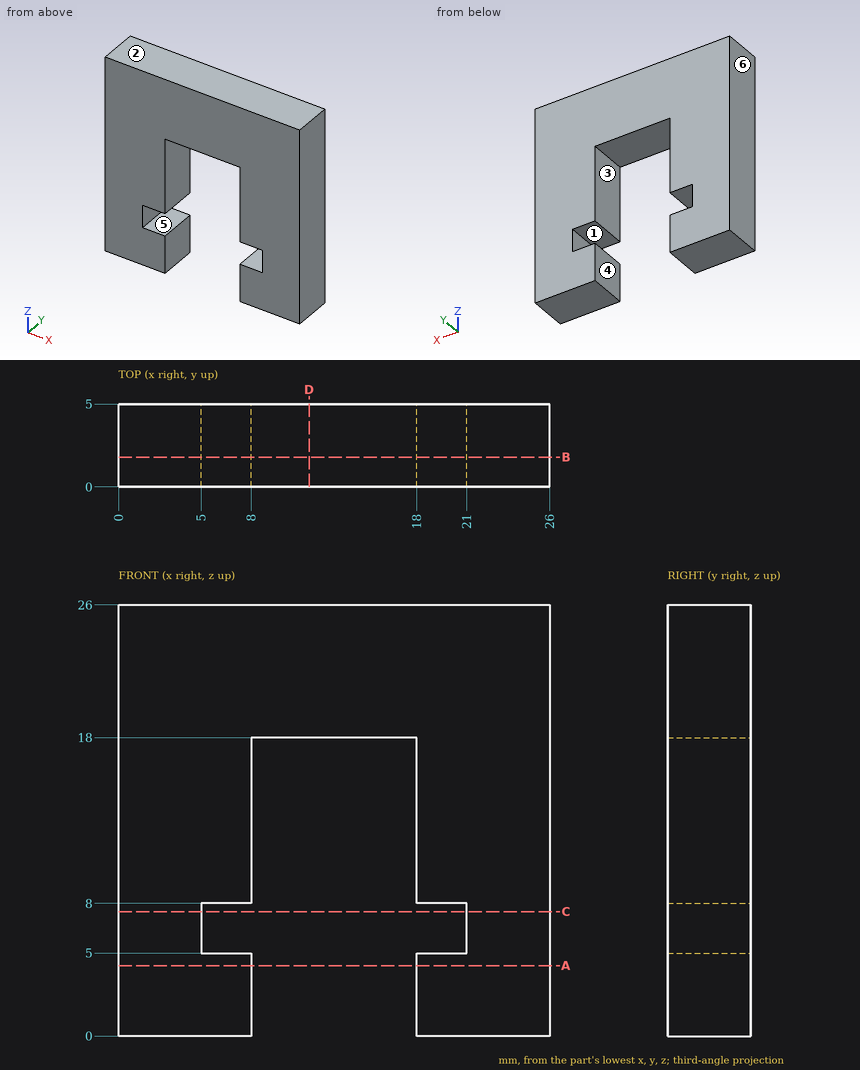
Geometry check sheet. Reference: drawing and pictorial views, mm from the part's lowest x, y, z. A direction names the side the tool comes from. Round coordinates to 2 decimals unless told otherwise and drop trailing zeros. Loops run counter-clockwise (first coordinate to the right, second up) from the corner with the lowest first, then second, coordinate; pieces in that order, holes last. Notation, with made-up numbers: M 46.25,-31 L 62.25,-31 A21 cw 62.25,-7 Z; hole C 12,89 d9. An arc over 180 degrees is marked long. Return JSON: item names as keys, results as strings. Group by question number.
(1) Section check B-B, the plane y = 1.8. Enter the section's corners in (x, z), and give its area (3 significant figures).
(2) Scan lines: line 1 along X through (y, z) = (0.7, 13.25); line 2 along X through (y, z) = (1.9, 6); line 3 along Z through (x, y) = (11, 0.2). Record each from-to range of solid material in increasing order. Write a range as [from, to].
(3) Section check A-A, the plane z = 4.25. Enter the section's corners in (x, y).
(4) Section check C-C, the plane z = 7.5. Enter the section's corners in (x, y), and give its area (3 significant figures).
(5) Set-up check for the marked faces 4, 5 and 6: record each of +Z, -Z, +X, -X, +Y, -Y from which the full face is reachable in a straight line by a thin tool's end or side.
(6) Go/stop test with a flat-tipped pin: pin 1 (1.5 mm diameter, centred on x = 12.5, y = 3, fed in from -Z). Record where the tip stops, or that it passes through.
(7) Section check D-D, the plane x = 11.5. Enter the section's corners in (y, z).
(8) Mould release check, pull along Z, two halves, no side actions. Record for the marked faces 1, 2 and 3: pulls with the +Z half, pulls with the -Z half, needs draft (parallel to the pull), parting line crosses it, or undercut.
Data:
{
 "1": {"outline": "M 0,0 L 8,0 L 8,5 L 5,5 L 5,8 L 8,8 L 8,18 L 18,18 L 18,8 L 21,8 L 21,5 L 18,5 L 18,0 L 26,0 L 26,26 L 0,26 Z", "area": "478 mm²"},
 "2": {"line 1": "[0, 8], [18, 26]", "line 2": "[0, 5], [21, 26]", "line 3": "[18, 26]"},
 "3": {"outline": "M 0,0 L 8,0 L 8,5 L 0,5 Z; M 18,0 L 26,0 L 26,5 L 18,5 Z"},
 "4": {"outline": "M 0,0 L 5,0 L 5,5 L 0,5 Z; M 21,0 L 26,0 L 26,5 L 21,5 Z", "area": "50.0 mm²"},
 "5": {"face 4": "-Z, +Y, -Y", "face 5": "+Y, -Y", "face 6": "+Z, -Z, -X, +Y, -Y"},
 "6": {"pin 1": "z = 18"},
 "7": {"outline": "M 0,18 L 5,18 L 5,26 L 0,26 Z"},
 "8": {"face 1": "undercut", "face 2": "pulls with the +Z half", "face 3": "needs draft"}
}
